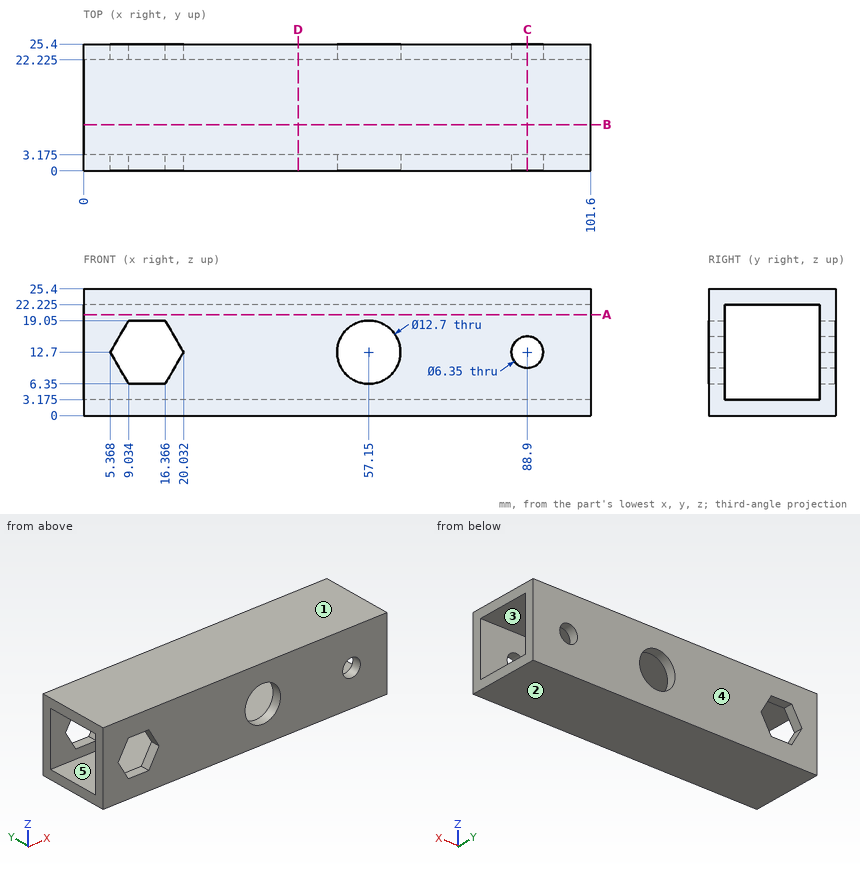
Answer from the drawing. Dimensions are ordinates in mm from the lowest x, y and z of the part. A direction names the side the tool comes from. Give positions to 0.01 mm unless a question says otherwise; leave off trailing zeros. Loops run counter-clockwise (first coordinate to the right, second up) from the corner with the lowest first, then second, coordinate; pieces in that order, holes last. Notation, with made-up numbers: (36, 36.25) - (73, 36.25) arc R11 cw to (73, 46.25) - close; hole circle Ø3 at (68, 66.25). An arc over 180 degrees is marked (long way). Answer as CSV lines item,"result". Start each with the question number.
Item 1: Find the intervals of material crossed by line 1 (X direction, y = 23.7, z = 12.7) (1 decimal); line 2 (Z direction, x = 88.9, y = 1.8) (1 decimal); line 3 (Y direction, x = 74.5, z = 8.25) (1 decimal), in increasing order. Write a range as from..to.
Item 2: This flat-tipped pin is pushed along its axis until it touches: pin 1 (7.5 mm diameter, centred on x = 57.15, z = 12.7, fed in from -Y). Where does it stop, or does it pass through?
Item 3: A cutting plane is placed at A-A on z = 20.25. Determine the outline of the cut face in (x, y) (1 decimal), then the cut area to 3 significant figures.
Item 4: A cutting plane is placed at C-C on x = 88.9. Determine the outline of the cut face in (y, z) (1 decimal), then the cut area to 3 significant figures.
Item 5: For the marked faces 4 and 5, determine the directions among +Z, -Z, +X, -X, +Y, -Y from which every point of the face is accessible in a straight line to the end or side of a thin tool.
Item 6: A cutting plane is placed at D-D on x = 43. Determine the outline of the cut face in (y, z) (1 decimal).
Item 7: The mould has two halves that part along Z. Classify the marked faces 1, 2 and 3: +Z half, -Z half, draft (parallel to the pull), parting line (faces both ways), or undercut.
Found:
1,line 1,"x = 0..5.4, 20..50.8, 63.5..85.7, 92.1..101.6"
1,line 2,"z = 0..9.5, 15.9..25.4"
1,line 3,"y = 0..3.2, 22.2..25.4"
2,pin 1,"passes through"
3,outline,"(0, 0) - (101.6, 0) - (101.6, 3.2) - (0, 3.2) - close; (0, 22.2) - (101.6, 22.2) - (101.6, 25.4) - (0, 25.4) - close"
3,area,"645 mm^2"
4,outline,"(0, 0) - (25.4, 0) - (25.4, 9.5) - (22.2, 9.5) - (22.2, 3.2) - (3.2, 3.2) - (3.2, 9.5) - (0, 9.5) - close; (0, 15.9) - (3.2, 15.9) - (3.2, 22.2) - (22.2, 22.2) - (22.2, 15.9) - (25.4, 15.9) - (25.4, 25.4) - (0, 25.4) - close"
4,area,"242 mm^2"
5,face 4,"+Z, -Z, +X, -X, +Y"
5,face 5,"+X, -X"
6,outline,"(0, 0) - (25.4, 0) - (25.4, 25.4) - (0, 25.4) - close; hole (3.2, 3.2) - (22.2, 3.2) - (22.2, 22.2) - (3.2, 22.2) - close"
7,face 1,"+Z half"
7,face 2,"-Z half"
7,face 3,"undercut"
